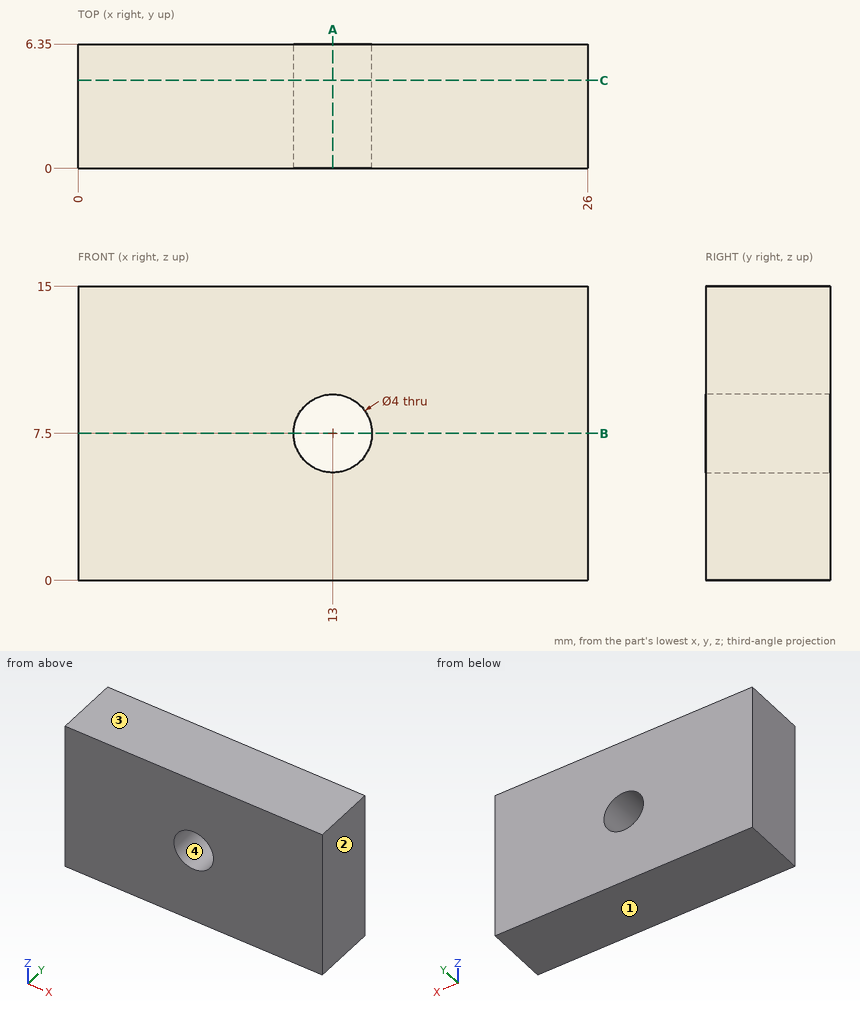
Input: dimensioned drawing with shaded views. Units: mm. Origin: part minimum x, y, z. Coordinates: 2 decimals unless noted, no trailing zeros. Loops run counter-clockwise (first coordinate to the right, second up) from the corner with the lowest first, then second, coordinate; pieces in that order, holes last. Notation, with made-up numbers: M -10.5,51.25 L 42.5,51.25 A15 cw 42.5,55.25 Z; hole C 39.5,26.5 d4. An arc over 180 degrees is marked long. Put each result on its own line as item: value.
(1) Cut plane A-A on x = 13. Return the cut outline in (y, z), then the cut area to 4 significant figures.
Answer sheet:
outline: M 0,0 L 6.35,0 L 6.35,5.5 L 0,5.5 Z; M 0,9.5 L 6.35,9.5 L 6.35,15 L 0,15 Z
area: 69.85 mm^2
(2) Cut plane C-C on y = 4.5. Return the cut outline in (x, z), then the cut area to 3 significant figures.
Answer sheet:
outline: M 0,0 L 26,0 L 26,15 L 0,15 Z; hole C 13,7.5 d4
area: 377 mm^2
(3) Material intervals for probe 1 along X at (y, z) = (3.5, 7.5); probe 2 along Z at (x, y) = (14.5, 5); probe 3 along X at (y, z) = (5, 8), sorted ascending.
Answer sheet:
probe 1: x = 0 to 11, 15 to 26
probe 2: z = 0 to 6.18, 8.82 to 15
probe 3: x = 0 to 11.06, 14.94 to 26
(4) Cut plane B-B on z = 7.5. Return the cut outline in (x, y), then the cut area to 3 significant figures.
Answer sheet:
outline: M 0,0 L 11,0 L 11,6.35 L 0,6.35 Z; M 15,0 L 26,0 L 26,6.35 L 15,6.35 Z
area: 140 mm^2
(5) Draft query along Z for the marked faces 1, 2, 3 and 4. Return one class per face: pulls with the +Z half, pulls with the -Z half, needs draft (parallel to the pull), parting line crosses it, or undercut.
Answer sheet:
face 1: pulls with the -Z half
face 2: needs draft
face 3: pulls with the +Z half
face 4: undercut
